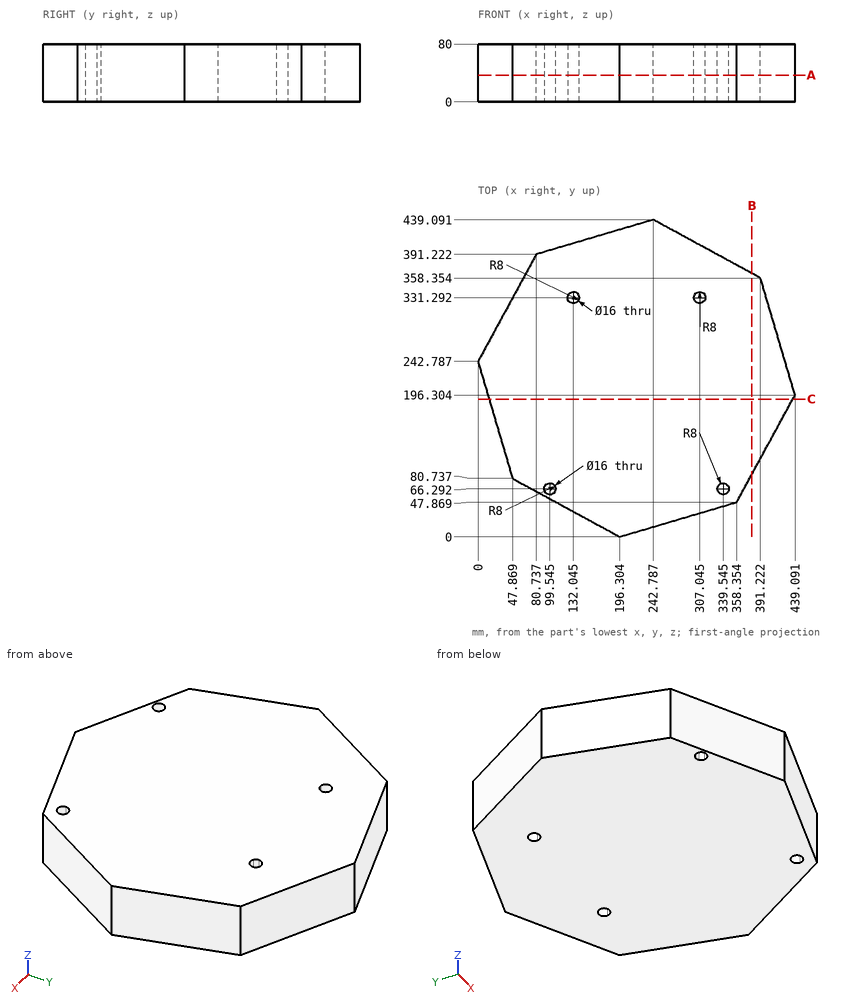
Study the drawing (mm; zero at the part's minimum x, y, z) and answer. Give positions to 0.01 mm unless a question says otherwise; leave off trailing zeros. Loops run counter-clockwise (first coordinate to the right, second up) from the corner with the lowest first, then second, coordinate; pieces in that order, holes last. Notation, with made-up numbers: M -15.75,23 L 8.25,23 A11 cw 8.25,29 Z; hole C 77.5,18.25 d3. An arc over 180 degrees is marked long. One line per item, written item: value. Start each with the question number.
1. Each of these flat-tipped pins is pushed along its axis until it touches: P1, Ø4, axis at x = 297, z = 17, coming from the +Y side; P2, Ø6, axis at y = 300, z = 37.5, coming from the +X side (1 decimal); P3, Ø6, axis at y = 72, z = 43, coming from the -X side (1 decimal). Where does it stop, or does it pass through?
2. Find the intervals of material crossed by probe 1 along Y at (x, z) = (125.5, 47.5) (1 decimal); probe 2 along Y at (x, z) = (172.5, 25.5); probe 3 along X at (y, z) = (85, 60), in increasing order.
3. Find section B-B (x = 379.5). Give the vertices of the cut face in (y, z), and give its area (3 significant figures).
4. Find section A-A (z = 37). Give the vertices of the cut face in (x, y) (1 decimal).
5. Find section C-C (y = 190.5). Give the vertices of the cut face in (x, z) (1 decimal).
Reported:
1. P1: stops at y = 410.69
1. P2: stops at x = 409.3
1. P3: stops at x = 58.4
2. probe 1: y = 38.5 to 326.7, 335.9 to 404.4
2. probe 2: y = 12.95 to 418.33
2. probe 3: x = 46.61 to 378.55
3. outline: M 86.75,0 L 364.73,0 L 364.73,80 L 86.75,80 Z
3. area: 22,200 mm²
4. outline: M 0,242.8 L 47.9,80.7 L 196.3,0 L 358.4,47.9 L 439.1,196.3 L 391.2,358.4 L 242.8,439.1 L 80.7,391.2 Z; hole C 99.5,66.3 d16; hole C 132,331.3 d16; hole C 307,331.3 d16; hole C 339.5,66.3 d16
5. outline: M 15.4,0 L 435.9,0 L 435.9,80 L 15.4,80 Z
